Could you check a few things on this drawing? It's one solid part, dimensions in mm from its lowest x, y, z. Coordinates: 2 decimals unless noted, no trailing zeros. Loops run counter-clockwise (first coordinate to the right, second up) from the corner with the lowest first, then second, coordinate; pieces in that order, holes last.
1) Imagine slicing it at B-B on y = 6.35. Please give me the cut outline in (x, z) (3 decimals), plus the area to 3 significant figures.
2) If I drill on line 1 along X through (y, z) = (6, 4.5); line 2 along Y through (x, z) = (76.2, 3.5) (3 decimals); line 3 along X through (y, z) = (8.5, 5.5), over which ranges is the centre line in solid material (lowest first)?
3) Will these pins go through, and if not, where does the flat tip stop? P1, Ø8.5, axis at x = 76.2, y = 6.35, coming from the -Z side; P2, Ø1.9, axis at x = 144, z = 1.5, coming from the +Y side; P3, Ø3.5, axis at y = 15.5, z = 1.5, coming from the -X side; P4, Ø3.5, axis at y = 15.5, z = 4, coming from the +X side.
4) Imagine slicing it at A-A on x = 101.6. Please give me the cut outline in (y, z) (3 decimals).
5) Imagine slicing it at C-C on z = 3.5. Give the number of separate pieces and of enclosed holes in the cut face, plus the area to 3 significant figures.
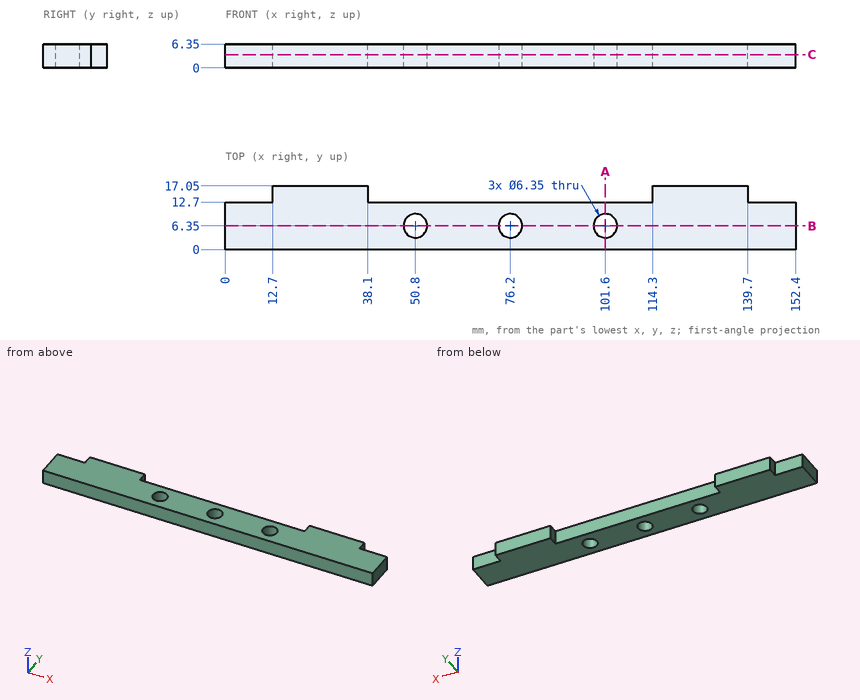
Filled in:
1. outline: (0, 0) - (47.625, 0) - (47.625, 6.35) - (0, 6.35) - close; (53.975, 0) - (73.025, 0) - (73.025, 6.35) - (53.975, 6.35) - close; (79.375, 0) - (98.425, 0) - (98.425, 6.35) - (79.375, 6.35) - close; (104.775, 0) - (152.4, 0) - (152.4, 6.35) - (104.775, 6.35) - close
1. area: 847 mm2
2. line 1: x = 0 to 47.64, 53.96 to 73.04, 79.36 to 98.44, 104.76 to 152.4
2. line 2: y = 0 to 3.175, 9.525 to 12.7
2. line 3: x = 0 to 48.46, 53.14 to 73.86, 78.54 to 99.26, 103.94 to 152.4
3. P1: stops at z = 0
3. P2: stops at y = 12.7
3. P3: stops at x = 12.7
3. P4: stops at x = 139.7
4. outline: (0, 0) - (3.175, 0) - (3.175, 6.35) - (0, 6.35) - close; (9.525, 0) - (12.7, 0) - (12.7, 6.35) - (9.525, 6.35) - close
5. separate pieces: 1
5. enclosed holes: 3
5. area: 2,060 mm2
